```python
from build123d import *

# Parameters (mm, degrees)
PAD_DEPTH    = 120
SKETCH001_R  = 1.75
PAD001_DEPTH = 3
FILLET_R     = 3


with BuildPart() as part:
    # Sketch → Pad (new body)
    with BuildSketch(Plane.XY):
        Polygon((0, 0), (79.5, 0), (79.5, 11), (77.5, 11), (77.5, 10), (78.5, 10), (78.5, 9), (77.5, 9), (77.5, 2), (55, 2), (55, 9), (54, 9), (54, 10), (55, 10), (55, 11), (51, 11), (51, 10), (52, 10), (52, 9), (51, 9), (51, 2), (28.5, 2), (28.5, 9), (27.5, 9), (27.5, 10), (28.5, 10), (28.5, 11), (24.5, 11), (24.5, 10), (25.5, 10), (25.5, 9), (24.5, 9), (24.5, 2), (2, 2), (2, 9), (1, 9), (1, 10), (2, 10), (2, 11), (0, 11), align=None)
    extrude(amount=PAD_DEPTH)

    # Sketch001 → Pad001 (join)
    with BuildSketch(Plane.XZ):
        Polygon((0, 6.726497), (-10, 12.5), (-10, 17.5), (0, 23.273503), align=None)
        with Locations((-5.25, 15)):
            Circle(SKETCH001_R, mode=Mode.SUBTRACT)
        Polygon((0, 66.726497), (-10, 72.5), (-10, 77.5), (0, 83.273503), align=None)
        with Locations((-5.25, 75)):
            Circle(SKETCH001_R, mode=Mode.SUBTRACT)
        Polygon((79.5, 36.726497), (89.5, 42.5), (89.5, 47.5), (79.5, 53.273503), align=None)
        with Locations((84.75, 45)):
            Circle(SKETCH001_R, mode=Mode.SUBTRACT)
        Polygon((79.5, 96.726497), (89.5, 102.5), (89.5, 107.5), (79.5, 113.273503), align=None)
        with Locations((84.75, 105)):
            Circle(SKETCH001_R, mode=Mode.SUBTRACT)
    extrude(amount=-PAD001_DEPTH)

    # Fillet
    fillet_edges = [part.edges().sort_by_distance(p)[0] for p in [
        (2, 2, 60),
        (28.5, 2, 60),
        (55, 2, 60),
        (24.5, 2, 60),
        (51, 2, 60),
        (77.5, 2, 60),
    ]]
    fillet(fillet_edges, radius=FILLET_R)


solid = part.part
```
Model file for the job. Use its own axes, mm. A direction names the side the tool comes from. Give positions to 0.01 mm unless a question says otherwise; leave off trailing zeros. Loops run counter-clockwise (first coordinate to the right, second up) from the corner with the lowest first, then second, coordinate; pieces in that order, holes last. Notation, with made-up numbers: M -11.75,72.5 L 46.25,72.5 A16 cw 46.25,79.5 Z; hole C -31.5,-39 d2. An arc over 180 degrees is marked long. Use one line per item in the form item = value.
Item 1: Slice it at B-B on x = 84.75. List the corners of the cut face in (y, z).
Filled in:
outline = M 0,39.76 L 3,39.76 L 3,43.25 L 0,43.25 Z; M 0,46.75 L 3,46.75 L 3,50.24 L 0,50.24 Z; M 0,99.76 L 3,99.76 L 3,103.25 L 0,103.25 Z; M 0,106.75 L 3,106.75 L 3,110.24 L 0,110.24 Z
Item 2: Which spindle directions (+Z, -Z, +X, -X, +Y, -Y) get a long thin tool onto all of the face, cutting with end or side? Do faces 1 (the flat face through (79.5, 5, 59)), 2 (the flat face through (82, 3, 45)), 3 (the flat face through (-5.07, 1.479, 20.346)), 4 (the flat face through (24.5, 7, 59)). Say none if no direction does.
Filled in:
face_1 = +X, +Y
face_2 = +Z, -Z, +X, +Y
face_3 = -X, +Y, -Y
face_4 = +Z, -Z, +Y
Item 3: Two-plate mould, pull along Z, no slides. Class faces 5 (the flat face through (-4.93, 1.479, 9.573)), 6 (the flat face through (2, 7, 59)), 7 (the flat face through (84.43, 1.479, 99.573)): released by +Z, released by -Z, zero draft, split by the parting line, or undercut.
Filled in:
face_5 = released by -Z
face_6 = zero draft
face_7 = undercut
Item 4: Drill centre lines: L1, parallel to X at y = 5.75, z = 102.5; L2, parallel to X at y = 0.75, z = 105; L3, parallel to Z at x = -5.25, y = 1.9. Where is each one in solid material? Low to high.
Filled in:
L1 = 0 to 2, 24.5 to 28.5, 51 to 55, 77.5 to 79.5
L2 = 0 to 83, 86.5 to 89.5
L3 = 9.76 to 13.25, 16.75 to 20.24, 69.76 to 73.25, 76.75 to 80.24
Item 5: Flat gauge pins, fed straight in: pin 1 Ø1 at (y, z) = (8, 31.5) entering from -X; pin 2 Ø3 at (x, z) = (83.5, 104.5) entering from +Y; pin 3 Ø0.5 at (y, z) = (9.5, 42) entering from +X. Where does each tip first touch, or does it go through?
Filled in:
pin_1 = 0
pin_2 = 3
pin_3 = 79.5
Item 6: Slice it at A-A on y = 6.75. List the corners of the cut face in (x, z), and give its area (3 significant figures).
Filled in:
outline = M 0,0 L 2,0 L 2,120 L 0,120 Z; M 24.5,0 L 28.5,0 L 28.5,120 L 24.5,120 Z; M 51,0 L 55,0 L 55,120 L 51,120 Z; M 77.5,0 L 79.5,0 L 79.5,120 L 77.5,120 Z
area = 1,440 mm^2
